Source: CAD feature listing. Evaluate the final solid. Frame: model axes, mm. A direction names the side the tool comes from. Round coordinates to 2 decimals unless told otherwise and drop trailing zeros. Write each loop counter-clockwise with the first axis right and the second up, starting at its lowest first coordinate (ties: lowest second). Pieces come first, ordered by that corner, then holes. Notation, with made-up numbers: M 78,28.5 L 120,28.5 A30 cw 120,67.5 Z; hole C 44,44 d5. An arc over 180 degrees is marked long. Use a Markdown table: item, result.
```python
from build123d import *

# Parameters (mm, degrees)
SKETCH3_W           = 70
SKETCH3_H           = 110
BOSS_EXTRUDE1_DEPTH = 3
SKETCH4_W           = 2.5
SKETCH4_H           = 105
BOSS_EXTRUDE2_DEPTH = 30
SKETCH5_R           = 3
BOSS_EXTRUDE3_DEPTH = 6
SKETCH7_W           = 70
SKETCH7_H           = 110
SKETCH7_W_2         = 65
SKETCH7_H_2         = 52.5
SKETCH7_H_3         = 50
BOSS_EXTRUDE4_DEPTH = 9.5
SKETCH8_W           = 15
SKETCH8_H           = 6
CUT_EXTRUDE2_DEPTH  = 2.5
SKETCH9_W           = 15
SKETCH9_H           = 15
CUT_EXTRUDE3_DEPTH  = 3
SKETCH10_W          = 1.5
SKETCH10_H          = 50
BOSS_EXTRUDE5_DEPTH = 9.5
SKETCH11_W          = 31
SKETCH11_H          = 2.5
CUT_EXTRUDE5_DEPTH  = 52.5
SKETCH12_R          = 3.5
BOSS_EXTRUDE6_DEPTH = 7
SKETCH15_R          = 1.5
CUT_EXTRUDE6_DEPTH  = 6
SKETCH16_W          = 65
SKETCH16_H          = 2.5
BOSS_EXTRUDE7_DEPTH = 52.5
SKETCH17_R          = 1.6
CUT_EXTRUDE7_DEPTH  = 95.942087611
SKETCH18_W          = 7
SKETCH18_H          = 3.7
CUT_EXTRUDE8_DEPTH  = 2.5
SKETCH19_R          = 1.5
CUT_EXTRUDE9_DEPTH  = 6
SKETCH20_R          = 10.5
CUT_EXTRUDE10_DEPTH = 2.5
FILLET2_R           = 2.5
FILLET3_R           = 2.5


with BuildPart() as part:
    # Sketch3 → Boss-Extrude1 (new body)
    with BuildSketch(Plane(origin=(0, 0, 0), x_dir=(1, 0, 0), z_dir=(0, 1, 0))):
        Rectangle(SKETCH3_W, SKETCH3_H)
    extrude(amount=BOSS_EXTRUDE1_DEPTH)

    # Sketch4 → Boss-Extrude2 (add)
    with BuildSketch(Plane(origin=(0, 3, 0), x_dir=(1, 0, 0), z_dir=(0, 1, 0))):
        with Locations((-33.75, 0)):
            Rectangle(SKETCH4_W, SKETCH4_H)
        Polygon((35, 55), (-35, 55), (-35, 52.5), (-32.5, 52.5), (32.5, 52.5), (35, 52.5), align=None)
        Polygon((35, -55), (35, 52.5), (32.5, 52.5), (32.5, -52.5), (32.5, -55), align=None)
        Polygon((-32.5, -52.5), (-35, -52.5), (-35, -55), (32.5, -55), (32.5, -52.5), align=None)
    extrude(amount=BOSS_EXTRUDE2_DEPTH)

    # Sketch5 → Boss-Extrude3 (add)
    with BuildSketch(Plane(origin=(0, 3, 0), x_dir=(1, 0, 0), z_dir=(0, 1, 0))):
        with Locations(Location((-24.06, 21.37, 0), (0, 0, 90))):
            Circle(SKETCH5_R)
        with Locations(Location((23.57, 21.37, 0), (0, 0, 90))):
            Circle(SKETCH5_R)
        with Locations(Location((23.57, -45.31, 0), (0, 0, 90))):
            Circle(SKETCH5_R)
        with Locations(Location((-24.06, -45.31, 0), (0, 0, 90))):
            Circle(SKETCH5_R)
    extrude(amount=BOSS_EXTRUDE3_DEPTH)

    # Sketch7 → Boss-Extrude4 (add)
    with BuildSketch(Plane.XZ):
        Rectangle(SKETCH7_W, SKETCH7_H)
        with Locations((0, -26.25)):
            Rectangle(SKETCH7_W_2, SKETCH7_H_2, mode=Mode.SUBTRACT)
        with Locations((0, 27.5)):
            Rectangle(SKETCH7_W_2, SKETCH7_H_3, mode=Mode.SUBTRACT)
    extrude(amount=BOSS_EXTRUDE4_DEPTH)

    # Sketch8 → Cut-Extrude2 (cut)
    with BuildSketch(Plane.XY.offset(2.5)):
        with Locations((17.5, -3)):
            Rectangle(SKETCH8_W, SKETCH8_H)
        with Locations((-17.5, -3)):
            Rectangle(SKETCH8_W, SKETCH8_H)
    extrude(amount=-CUT_EXTRUDE2_DEPTH, mode=Mode.SUBTRACT)

    # Sketch9 → Cut-Extrude3 (cut)
    with BuildSketch(Plane.XZ):
        with Locations((-17.5, -7.5)):
            Rectangle(SKETCH9_W, SKETCH9_H)
        with Locations((17.5, -7.5)):
            Rectangle(SKETCH9_W, SKETCH9_H)
    extrude(amount=-CUT_EXTRUDE3_DEPTH, mode=Mode.SUBTRACT)

    # Sketch10 → Boss-Extrude5 (add)
    with BuildSketch(Plane.XZ):
        with Locations((-31.75, 27.5)):
            Rectangle(SKETCH10_W, SKETCH10_H)
        with Locations((31.75, 27.5)):
            Rectangle(SKETCH10_W, SKETCH10_H)
    extrude(amount=BOSS_EXTRUDE5_DEPTH)

    # Sketch11 → Cut-Extrude5 (cut)
    with BuildSketch(Plane.XY.offset(55)):
        with Locations((-15.5, -8.25)):
            Rectangle(SKETCH11_W, SKETCH11_H)
        Polygon((-33.5, -7), (-31, -9.5), (-31, -7), align=None)
        with Locations((15.5, -8.25)):
            Rectangle(SKETCH11_W, SKETCH11_H)
        Polygon((31, -7), (31, -9.5), (33.5, -7), align=None)
    extrude(amount=-CUT_EXTRUDE5_DEPTH, mode=Mode.SUBTRACT)

    # Sketch12 → Boss-Extrude6 (add)
    with BuildSketch(Plane.XZ):
        with Locations(Location((0, 48, 0), (0, 0, 270))):
            Circle(SKETCH12_R)
    extrude(amount=BOSS_EXTRUDE6_DEPTH)

    # Sketch15 → Cut-Extrude6 (cut)
    with BuildSketch(Plane.XZ.offset(7)):
        with Locations(Location((0, 48, 0), (0, 0, 270))):
            Circle(SKETCH15_R)
    extrude(amount=-CUT_EXTRUDE6_DEPTH, mode=Mode.SUBTRACT)

    # Sketch16 → Boss-Extrude7 (add)
    with BuildSketch(Plane.XY.offset(-52.5)):
        with Locations((0, -8.25)):
            Rectangle(SKETCH16_W, SKETCH16_H)
    extrude(amount=BOSS_EXTRUDE7_DEPTH)

    # Sketch17 → Cut-Extrude7 (cut, through all)
    with BuildSketch(Plane.ZY.offset(35)):
        with Locations((-37.5, 28)):
            Circle(SKETCH17_R)
        with Locations((37.5, 28)):
            Circle(SKETCH17_R)
    extrude(amount=-CUT_EXTRUDE7_DEPTH, mode=Mode.SUBTRACT)

    # Sketch18 → Cut-Extrude8 (cut)
    with BuildSketch(Plane(origin=(0, 0, -55), x_dir=(-1, 0, 0), z_dir=(0, 0, -1))):
        with Locations((0, 5.85)):
            Rectangle(SKETCH18_W, SKETCH18_H)
    extrude(amount=-CUT_EXTRUDE8_DEPTH, mode=Mode.SUBTRACT)

    # Sketch19 → Cut-Extrude9 (cut)
    with BuildSketch(Plane(origin=(0, 9, 0), x_dir=(1, 0, 0), z_dir=(0, 1, 0))):
        with Locations(Location((-24.06, -45.31, 0), (0, 0, 270))):
            Circle(SKETCH19_R)
        with Locations(Location((-24.06, 21.37, 0), (0, 0, 270))):
            Circle(SKETCH19_R)
        with Locations(Location((23.57, 21.37, 0), (0, 0, 270))):
            Circle(SKETCH19_R)
        with Locations(Location((23.57, -45.31, 0), (0, 0, 270))):
            Circle(SKETCH19_R)
    extrude(amount=-CUT_EXTRUDE9_DEPTH, mode=Mode.SUBTRACT)

    # Sketch20 → Cut-Extrude10 (cut)
    with BuildSketch(Plane(origin=(0, 0, -55), x_dir=(-1, 0, 0), z_dir=(0, 0, -1))):
        with Locations((-19.5, 17.5)):
            Circle(SKETCH20_R)
    extrude(amount=-CUT_EXTRUDE10_DEPTH, mode=Mode.SUBTRACT)

    # Fillet2
    # the kernel refuses this fillet: 2.5 mm, written as the material it takes off along each edge
    with BuildSketch(Plane(origin=(-35, -15.75, -55), x_dir=(1, 0, 0), z_dir=(0, 1, 0)), Plane(origin=(35, 39.25, -55), x_dir=(-1, 0, 0), z_dir=(0, -1, 0)), Plane(origin=(35, 39.25, 55), x_dir=(0, 0, -1), z_dir=(0, -1, 0)), Plane(origin=(-35, -15.75, 55), x_dir=(0, 0, -1), z_dir=(0, 1, 0))) as fillet2_piece_1:
        with BuildLine():
            CenterArc((FILLET2_R, -FILLET2_R), FILLET2_R, 90, 90)
            Line((0, -FILLET2_R), (0, 0))
            Line((0, 0), (FILLET2_R, 0))
        make_face()
    extrude(amount=55, mode=Mode.SUBTRACT)

    # Fillet3
    # the kernel refuses this fillet: 2.5 mm, written as the material it takes off along each edge
    with BuildSketch(Plane(origin=(-32.5, -9.5, -52.5), x_dir=(-1, 0, 0), z_dir=(0, 0, 1))) as fillet3_piece_1:
        with BuildLine():
            CenterArc((2.5 - FILLET3_R, -FILLET3_R), FILLET3_R, 0, 90)
            Line((2.5, -FILLET3_R), (2.5, 0))
            Line((2.5, 0), (2.5 - FILLET3_R, 0))
        make_face()
    revolve(axis=Axis((-32.5, -9.5, -52.5), (0, -1, 0)), revolution_arc=90, mode=Mode.SUBTRACT)
    with BuildSketch(Plane(origin=(32.5, -9.5, -52.5), x_dir=(1, 0, 0), z_dir=(0, 0, 1))) as fillet3_piece_2:
        with BuildLine():
            CenterArc((2.5 - FILLET3_R, FILLET3_R), FILLET3_R, 270, 90)
            Line((2.5 - FILLET3_R, 0), (2.5, 0))
            Line((2.5, 0), (2.5, FILLET3_R))
        make_face()
    revolve(axis=Axis((32.5, -9.5, -52.5), (0, 1, 0)), revolution_arc=90, mode=Mode.SUBTRACT)
    with BuildSketch(Plane(origin=(35, -9.5, -52.5), x_dir=(-1, 0, 0), z_dir=(0, 0, 1)), Plane(origin=(-35, -9.5, 58.75), x_dir=(1, 0, 0), z_dir=(0, 0, -1))) as fillet3_piece_3:
        with BuildLine():
            CenterArc((FILLET3_R, -FILLET3_R), FILLET3_R, 90, 90)
            Line((0, -FILLET3_R), (0, 0))
            Line((0, 0), (FILLET3_R, 0))
        make_face()
    extrude(amount=111.25, mode=Mode.SUBTRACT)
    with BuildSketch(Plane(origin=(-32.5, -9.5, -55), x_dir=(0, 1, 0), z_dir=(1, 0, 0))) as fillet3_piece_4:
        with BuildLine():
            CenterArc((FILLET3_R, FILLET3_R), FILLET3_R, 180, 90)
            Line((0, FILLET3_R), (0, 0))
            Line((0, 0), (FILLET3_R, 0))
        make_face()
    extrude(amount=65, mode=Mode.SUBTRACT)


solid = part.part
```
Q1. First-contact query: pin 1 Ø6 at (x, z) = (7, -7) entering from +Y; pin 2 Ø1.9 at (y, z) = (28, -37.5) entering from -X; pin 3 Ø1.8 at (x, z) = (-24.06, 45.31) entering from -Y; pin 4 Ø5.5 at (x, z) = (1, 46.5) entering from -Y. Flat tips, straight axial feed; report the tip coordinate or a pass-through.
Results are:
| item | result |
|---|---|
| pin 1 | y = 3 |
| pin 2 | through |
| pin 3 | y = 0 |
| pin 4 | y = -7 |
Q2. Section B-B on y = -3. Return loops of the section in (x, z).
Results are:
| item | result |
|---|---|
| outline | M -35,-52.5 A2.5 ccw -32.5,-55 L 32.5,-55 A2.5 ccw 35,-52.5 L 35,52.5 A2.5 ccw 32.5,55 L -32.5,55 A2.5 ccw -35,52.5 Z; M -10,0 L 10,0 L 10,2.5 L -10,2.5 Z; C 0,48 d7; hole M -32.5,-52.5 L 32.5,-52.5 L 32.5,0 L 25,0 L 25,2.5 L 31,2.5 L 31,52.5 L -31,52.5 L -31,2.5 L -25,2.5 L -25,0 L -32.5,0 Z; hole C 0,48 d3 |
Q3. Line query: L1, parallel to Z at x = 8.5, y = -1; L2, parallel to X at y = 7.35, z = 45.31; L3, parallel to X at y = -4, z = -16. Output: solid intervals per line, ascending.
Results are:
| item | result |
|---|---|
| L1 | -55 to -52.5, 0 to 2.5, 52.5 to 55 |
| L2 | -35 to -32.5, -27.06 to -25.56, -22.56 to -21.06, 20.57 to 22.07, 25.07 to 26.57, 32.5 to 35 |
| L3 | -35 to -32.5, 32.5 to 35 |
Q4. Mould query, pull axis X, two halves, no side actions, for faces 1 (the flat face through (0, -3, 52.5)), 2 (the cylindrical face through (-34, -9, 2)), 3 (the cylindrical face through (33.732, 29.586, -37.708)). Classes: +X half, -X half, draft (parallel to the pull), parting line (faces both ways), or undercut.
Results are:
| item | result |
|---|---|
| face 1 | undercut |
| face 2 | -X half |
| face 3 | draft |
Q5. Section C-C on z = 37.5. Return loops of the section in (x, y).
Results are:
| item | result |
|---|---|
| outline | M -35,-7 A2.5 ccw -32.5,-9.5 L -31,-9.5 L -33.5,-7 L -31,-7 L -31,0 L 31,0 L 31,-7 L 33.5,-7 L 31,-9.5 L 32.5,-9.5 A2.5 ccw 35,-7 L 35,26.4 L 32.5,26.4 L 32.5,3 L -32.5,3 L -32.5,26.4 L -35,26.4 Z; M -35,29.6 L -32.5,29.6 L -32.5,33 L -35,33 Z; M 32.5,29.6 L 35,29.6 L 35,33 L 32.5,33 Z |
Q6. Section D-D on z = -4. Return loops of the section in (x, y), plus the area to 3 significant figures.
Results are:
| item | result |
|---|---|
| outline | M -35,-7 A2.5 ccw -32.5,-9.5 L 32.5,-9.5 A2.5 ccw 35,-7 L 35,33 L 32.5,33 L 32.5,3 L 25,3 L 25,0 L 32.5,0 L 32.5,-7 L -32.5,-7 L -32.5,0 L -25,0 L -25,3 L -32.5,3 L -32.5,33 L -35,33 Z; M -10,0 L 10,0 L 10,3 L -10,3 Z |
| area | 477 mm^2 |
Q7. Section A-A on x = 0. Give the number of separate pieces and of enclosed holes in the cut face, plus the area to 3 significant figures.
Results are:
| item | result |
|---|---|
| separate pieces | 2 |
| enclosed holes | 1 |
| area | 697 mm^2 |
Q8. Reachability of faces 4 (the flat face through (31, -3, 27)), 5 (the flat face through (-34, 33, 0)), 6 (the flat face through (32.5, 18, -1)), 7 (the cylindrical face through (-34.248, 12.72, -54.287)), 8 (the flat face through (-25, -3, 1)) from +Z, -Z, +X, -X, +Y, -Y: full face, straight path, thin tool, end or side. Return the list, or none.
Results are:
| item | result |
|---|---|
| face 4 | -Y |
| face 5 | +Z, -Z, +X, -X, +Y |
| face 6 | +Y |
| face 7 | -Z, -X, +Y, -Y |
| face 8 | none |
